Build history of the part. All positions in model axes, mm. A direction names the side the tool comes from. Round coordinates to 2 decimals unless told otherwise and drop trailing zeros. Write each loop counter-clockwise with the first axis right and the second up, starting at its lowest first coordinate (ties: lowest second). Pieces come first, ordered by that corner, then holes. Notation, with made-up numbers: M 7.5,72 L 16.5,72 A25 ccw 16.5,88 Z; hole C 79.25,5 d7. An arc over 180 degrees is marked long. Write item = value, one per line. Start each with the question number.
Q1. Band-saw the part on A-A on y = -21.5. Write the cut outline in (x, z).
Q2. Tool access for faces 1 (the flat face through (-5, -21, 894)), 2 (the flat face through (0, -17, 894)): list every direction of +Z, -Z, +X, -X, +Y, -Y with a clear straight run to the whole face (end or side of a thin tool).
Q3. Band-saw the part on B-B on z = 824. Write the cut outline in (x, y), plus the area to 3 significant figures.
Q4. Drop flat-ended pins along their axis: P1, Ø15, axis at y = -21, z = 142, coming from the -X side; P2, Ø2.5, axis at x = -2, y = -24.5, coming from the +Z side; P3, Ø5, axis at x = -27.5, z = 151.5, coming from the -Y side. Give the stop position or say it passes through.
Q5. Band-saw the part on C-C on z = 696.5. Write the cut outline in (x, y).
Q6. Probe L1, parallel to Z at x = -56, y = -3.5; L2, parallel to X at y = -12.5, z = 188.5. List the from-to ranges inside material, lowest first.
```python
from build123d import *

# Parameters (mm, degrees)
F1_DEPTH = 5
F3_W     = 5
F3_H     = 229.9418896437
F3_H_2   = 160
F4_DEPTH = 35
F6_R     = 5
F7_DEPTH = 8


with BuildPart() as f1:
    # F0 (on Front) → F1 (new body)
    with BuildSketch(Plane.XZ):
        Polygon((-70, 0), (0, 0), (0, 230), (-40, 230), (-40, 815), (0, 815), (0, 975), (-70, 975), align=None)
        with BuildLine():
            ThreePointArc((-59, 108), (-55, 112), (-51, 108))
            Line((-51, 108), (-51, 8))
            ThreePointArc((-51, 8), (-55, 4), (-59, 8))
            Line((-59, 8), (-59, 108))
        make_face(mode=Mode.SUBTRACT)
        with BuildLine():
            ThreePointArc((-29, 212), (-25, 216), (-21, 212))
            Line((-21, 212), (-21, 8))
            ThreePointArc((-21, 8), (-25, 4), (-29, 8))
            Line((-29, 8), (-29, 212))
        make_face(mode=Mode.SUBTRACT)
        with BuildLine():
            ThreePointArc((-59, 963), (-55, 967), (-51, 963))
            Line((-51, 963), (-51, 863))
            ThreePointArc((-51, 863), (-55, 859), (-59, 863))
            Line((-59, 863), (-59, 963))
        make_face(mode=Mode.SUBTRACT)
    extrude(amount=F1_DEPTH)

    # F3 (on offset) → F4 (join)
    with BuildSketch(Plane(origin=(0, 0, 0), x_dir=(-1, 0, 0), z_dir=(0, 1, 0))):
        with Locations((2.5, 114.9709448218)):
            Rectangle(F3_W, F3_H)
        with Locations((2.5, 894.9537706375)):
            Rectangle(F3_W, F3_H_2)
    extrude(amount=-F4_DEPTH)

    # F6 (on offset) → F7 (join)
    with BuildSketch(Plane.XZ.offset(5)):
        with Locations((-55.5474348366, 48)):
            Circle(F6_R)
        with Locations((-24.9165232928, 183)):
            Circle(F6_R)
        with Locations((-25.0249505043, 196)):
            Circle(F6_R)
    extrude(amount=-F7_DEPTH)


solid = f1.part
```
Conclusion:
q1.outline = M -5,0 L 0,0 L 0,229.94 L -5,229.94 Z; M -5,814.95 L 0,814.95 L 0,974.95 L -5,974.95 Z
q2.face_1 = +Z, -Z, -X, -Y
q2.face_2 = +Z, -Z, +X, +Y, -Y
q3.outline = M -70,-5 L -5,-5 L -5,-35 L 0,-35 L 0,0 L -70,0 Z
q3.area = 500 mm^2
q4.P1 = -5
q4.P2 = 974.95
q4.P3 = -5
q5.outline = M -70,-5 L -40,-5 L -40,0 L -70,0 Z
q6.L1 = 0 to 4.13, 43.02 to 52.98, 111.87 to 859.13, 966.87 to 975
q6.L2 = -5 to 0
